Geometry: final body of the model. Coordinates: model frame, mm. Face numbers are marked on the shaded views. A direction names the side the tool comes from. Give positions to 0.01 mm unless a question says otherwise; leave off trailing zeros. Order: outer loops, then holes, each group sorted by start corner. A loop starts at its lowest first (then second) coordinate and runs counter-clockwise, first axis right, second up. Notation, with made-up numbers: (85, 38) - (118, 38) arc R34 cw to (118, 74) - close; hole circle Ø10 at (74.5, 83.5). An arc over 180 degrees is marked (long way). Use one line per item in the form item = value.
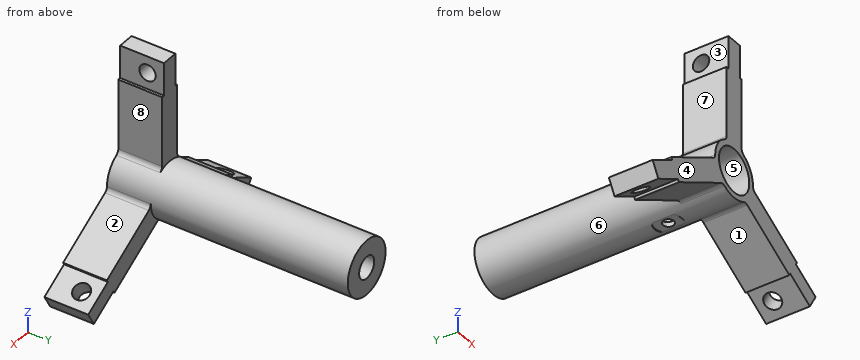
from build123d import *

# Parameters (mm, degrees)
BOSS_EXTRUDE1_REACH      = 170.065
BOSS_EXTRUDE1_END_RADIUS = 15.875
SKETCH2_W                = 9.525
SKETCH2_H                = 25.4
SKETCH3_R                = 4.7625
CUT_EXTRUDE1_DEPTH       = 161.463193307
BOSS_EXTRUDE2_REACH      = 160.432
BOSS_EXTRUDE2_END_RADIUS = 15.875
SKETCH4_W                = 12.7
SKETCH4_H                = 25.4
FILLET1_R                = 3.175
CIRPATTERN1_COUNT        = 3
FILLET1_OF_CIRPATTERN1_R = 3.175
SKETCH5_R                = 7.9375
CUT_EXTRUDE3_DEPTH       = 0.635
SKETCH6_R                = 3.175
CUT_EXTRUDE4_DEPTH       = 12.7


with BuildPart() as part:
    # Sketch1 → Base-Revolve (revolve)
    with BuildSketch(Plane.XY, mode=Mode.PRIVATE) as base_revolve_sk:
        Polygon((12.7, 0), (12.7, 127), (6.35, 127), (6.35, 139.7), (15.875, 139.7), (15.875, 0), align=None)
    revolve(base_revolve_sk.sketch.rotate(Axis((0, 118.223731343, 0), (0, -1, 0)), 90), axis=Axis((0, 118.223731343, 0), (0, -1, 0)))

    # Boss-Extrude1: up to this cylinder (the profile starts outside it)
    boss_extrude1_end = Plane(origin=(0, 12.7, 0), z_dir=(0, 1, 0)) * Cylinder(BOSS_EXTRUDE1_END_RADIUS, 372.88, mode=Mode.PRIVATE)
    # Sketch2 → Boss-Extrude1 (add, up to the surface)
    with BuildSketch(Plane.XY.offset(76.2), mode=Mode.PRIVATE) as boss_extrude1_sk1:
        with Locations((0, 12.7)):
            Rectangle(SKETCH2_W, SKETCH2_H)
    boss_extrude1_tool1 = extrude(boss_extrude1_sk1.sketch, amount=-BOSS_EXTRUDE1_REACH, mode=Mode.PRIVATE) - boss_extrude1_end
    boss_extrude1 = boss_extrude1_tool1.solids().sort_by_distance((0, 12.7, 76.2))[0]
    add(boss_extrude1)

    # Sketch3 → Cut-Extrude1 (cut, through all)
    with BuildSketch(Plane(origin=(4.7625, 0, 0), x_dir=(0, 0, -1), z_dir=(1, 0, 0))):
        with Locations((-66.675, 15.875)):
            Circle(SKETCH3_R)
    cut_extrude1 = extrude(amount=-CUT_EXTRUDE1_DEPTH, mode=Mode.SUBTRACT)

    # Boss-Extrude2: up to this cylinder (the profile starts outside it)
    boss_extrude2_end = Plane(origin=(0, 12.7, 0), z_dir=(0, 1, 0)) * Cylinder(BOSS_EXTRUDE2_END_RADIUS, 353.614, mode=Mode.PRIVATE)
    # Sketch4 → Boss-Extrude2 (add, up to the surface)
    with BuildSketch(Plane.XY.offset(57.15), mode=Mode.PRIVATE) as boss_extrude2_sk1:
        with Locations((0, 12.7)):
            Rectangle(SKETCH4_W, SKETCH4_H)
    boss_extrude2_tool1 = extrude(boss_extrude2_sk1.sketch, amount=-BOSS_EXTRUDE2_REACH, mode=Mode.PRIVATE) - boss_extrude2_end
    boss_extrude2 = boss_extrude2_tool1.solids().sort_by_distance((0, 12.7, 57.15))[0]
    add(boss_extrude2)

    # Fillet1
    fillet1_edges = [part.edges().sort_by_distance(p)[0] for p in [
        (-6.35, 12.7, 14.549677831),
        (6.35, 12.7, 14.549677831),
    ]]
    fillet(fillet1_edges, radius=FILLET1_R)

    # CirPattern1: Boss-Extrude1, Cut-Extrude1, Boss-Extrude2 ×3 about axis
    cirpattern1_axis = Axis((0, 0, 0), (0, 1, 0))
    add([boss_extrude1.rotate(cirpattern1_axis, i * 360 / CIRPATTERN1_COUNT) for i in range(1, CIRPATTERN1_COUNT)])
    add([cut_extrude1.rotate(cirpattern1_axis, i * 360 / CIRPATTERN1_COUNT) for i in range(1, CIRPATTERN1_COUNT)], mode=Mode.SUBTRACT)
    add([boss_extrude2.rotate(cirpattern1_axis, i * 360 / CIRPATTERN1_COUNT) for i in range(1, CIRPATTERN1_COUNT)])

    # Fillet1 of CirPattern1
    fillet1_of_cirpattern1_edges = [part.edges().sort_by_distance(p)[0] for p in [
        (15.775390619, 12.7, -1.775577602),
        (9.425390619, 12.7, -12.77410023),
        (-9.425390619, 12.7, -12.77410023),
        (-15.775390619, 12.7, -1.775577602),
    ]]
    fillet(fillet1_of_cirpattern1_edges, radius=FILLET1_OF_CIRPATTERN1_R)

    # Sketch5 → Cut-Extrude3 (cut)
    with BuildSketch(Plane.XY.offset(-15.875)):
        with Locations((0, 38.1)):
            Circle(SKETCH5_R)
    extrude(amount=CUT_EXTRUDE3_DEPTH, mode=Mode.SUBTRACT)

    # Sketch6 → Cut-Extrude4 (cut)
    with BuildSketch(Plane(origin=(0, 0, -15.24), x_dir=(-1, 0, 0), z_dir=(0, 0, -1))):
        with Locations((0, 38.1)):
            Circle(SKETCH6_R)
    extrude(amount=-CUT_EXTRUDE4_DEPTH, mode=Mode.SUBTRACT)


solid = part.part
(1) Ray query, line 1 along X through (y, z) = (78, 0) (3 decimals); line 2 along Y through (x, z) = (4.5, 30.5); line 3 along Y through (x, z) = (0, -14) (3 decimals). Return the intervals inside material, ascending.
Computed values:
line_1 = -15.875 to -12.7, 12.7 to 15.875
line_2 = 0 to 25.4
line_3 = 0 to 34.925, 41.275 to 139.7
(2) Cut plane C-C on z = 45.5. Output: boundary loops of the cut face in (x, y).
Computed values:
outline = (-6.35, 0) - (6.35, 0) - (6.35, 25.4) - (-6.35, 25.4) - close
(3) Pull-direction query (X, two-part tool) for the marked faces 1, 2, 3 and 4; classes: released by +X, released by -X, zero draft, split by the parting line, or undercut.
Computed values:
face_1 = undercut
face_2 = released by +X
face_3 = released by -X
face_4 = zero draft
(4) Cut plane A-A on x = 0. Give the number of separate pieces and of enclosed holes in the cut face, plus the area to 3 significant figures.
Computed values:
separate_pieces = 3
enclosed_holes = 1
area = 2,480 mm²
(5) Reachability of the marked faces 5, 6, 7 and 8 from +Z, -Z, +X, -X, +Y, -Y: full face, straight path, thin tool, end or side. Return the list, or none.
Computed values:
face_5 = -Y
face_6 = +Y
face_7 = +Z, -X, +Y, -Y
face_8 = +Z, +X, +Y, -Y
(6) Cut plane D-D on y = 116. Output: boundary loops of the cut face in (x, z) (3 decimals).
Computed values:
outline = circle Ø31.75 at (0, 0); hole circle Ø25.4 at (0, 0)
(7) Contact query for flat-ended pins moving along their axis: pin 1 Ø20.5 at (y, z) = (10, 33) entering from +X; pin 2 Ø1.5 at (x, y) = (-13, 43) entering from +Z; pin 3 Ø5.5 at (y, z) = (14, 70.5) entering from +X. Output: stop coordinate, or through.
Computed values:
pin_1 = 6.35
pin_2 = 10.1
pin_3 = 4.76
(8) Cut plane B-B on y = 38.1. Output: boundary loops of the cut face in (x, z) (3 decimals), plus the area to 3 significant figures.
Computed values:
outline = (-4.445, -15.24) - (-3.175, -15.24) - (-3.175, -12.297) arc R12.7 cw (long way) to (3.175, -12.297) - (3.175, -15.24) - (4.445, -15.24) arc R15.875 ccw (long way) to start
area = 264 mm²
